The figure shows three views and two pictorial views of one solid part (mm, origin at its lowest corner). Answer the questions. Coordinates: 2 decimals unless noted, no trailing zeros. Write each loop counter-clockwise with the first axis right and the second up, starting at its lowest first coordinate (ties: lowest second). Pieces come first, ordered by that corner, then holes.
Item 1: This flat-tipped pin is pushed along its axis until it touches: P1, Ø1, axis at y = 18, z = 1, coming from the -X side. Where does it stop, or does it pass through?
Item 2: Section A-A (y = 37) is taken. Give the vertices of the cut face in (x, z), then the cut area to 3 significant figures.
Item 3: Straight lines are drawn through the part: probe 1 along Y at (x, z) = (1.5, 0.25); probe 2 along Z at (x, y) = (2.1, 11); probe 3 along X at (y, z) = (20.5, 3.2). For each, find the intervals that lie inside material, in ascending order.
Item 4: Section C-C (z = 2.5) is taken. Give the vertices of the cut face in (x, y), then the cut area to 3 significant figures.
Item 5: Section B-B (x = 1.7) is taken. Give the vertices of the cut face in (y, z).
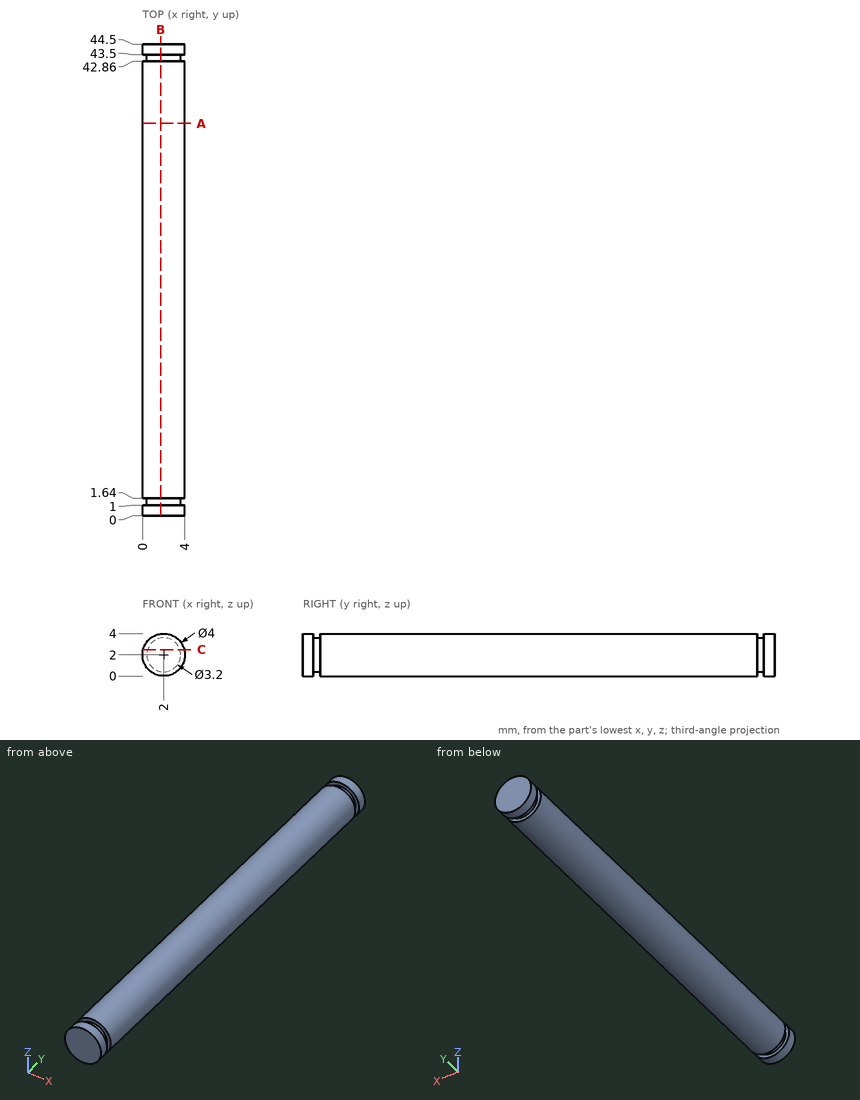
Established:
1. P1: stops at x = 0.06
2. outline: circle Ø4 at (2, 2)
2. area: 12.6 mm2
3. probe 1: y = 0 to 1, 1.64 to 42.86, 43.5 to 44.5
3. probe 2: z = 0 to 4
3. probe 3: x = 0.4 to 3.6
4. outline: (0.06, 0) - (3.94, 0) - (3.94, 1) - (3.52, 1) - (3.52, 1.64) - (3.94, 1.64) - (3.94, 42.86) - (3.52, 42.86) - (3.52, 43.5) - (3.94, 43.5) - (3.94, 44.5) - (0.06, 44.5) - (0.06, 43.5) - (0.48, 43.5) - (0.48, 42.86) - (0.06, 42.86) - (0.06, 1.64) - (0.48, 1.64) - (0.48, 1) - (0.06, 1) - close
4. area: 171 mm2
5. outline: (0, 0.02) - (1, 0.02) - (1, 0.43) - (1.64, 0.43) - (1.64, 0.02) - (42.86, 0.02) - (42.86, 0.43) - (43.5, 0.43) - (43.5, 0.02) - (44.5, 0.02) - (44.5, 3.98) - (43.5, 3.98) - (43.5, 3.57) - (42.86, 3.57) - (42.86, 3.98) - (1.64, 3.98) - (1.64, 3.57) - (1, 3.57) - (1, 3.98) - (0, 3.98) - close
